Could you check a few things on this model? Use its own coordinates, in mm. A direction names the side the tool comes from. Round coordinates to 2 decimals unless told otherwise and drop trailing zeros. Write each loop counter-clockwise with the first axis right and the second up, starting at its lowest first coordinate (ties: lowest second). Pieces come first, ordered by that corner, then holes.
```python
from build123d import *

# Parameters (mm, degrees)
SKETCH_1_R          = 1.5
EXTRUDE_1_DEPTH     = 3
FILLET_1_R          = 2
SKETCH_3_W          = 25.138692766
SKETCH_3_H          = 29.703861026
CUT_EXTRUDE_1_DEPTH = 38.353045391
SKETCH_4_W          = 21
SKETCH_4_H          = 34
EXTRUDE_2_DEPTH     = 3
SKETCH_5_W          = 7
SKETCH_5_H          = 54
CUT_EXTRUDE_2_DEPTH = 50.226517244
FILLET_2_R          = 1


with BuildPart() as part:
    # 草图1 → 凸台-拉伸1 (new body)
    with BuildSketch(Plane.XY):
        Polygon((-10.5, 14), (10.5, 14), (10.5, 4), (34.5, 4), (34.5, -4), (10.5, -4), (10.5, -14), (-10.5, -14), align=None)
        with Locations((-7.5, 5)):
            Circle(SKETCH_1_R, mode=Mode.SUBTRACT)
        with Locations((7.5, 5)):
            Circle(SKETCH_1_R, mode=Mode.SUBTRACT)
        with Locations((-7.5, -5)):
            Circle(SKETCH_1_R, mode=Mode.SUBTRACT)
        with Locations((7.5, -5)):
            Circle(SKETCH_1_R, mode=Mode.SUBTRACT)
        with Locations((16.5, 0)):
            Circle(SKETCH_1_R, mode=Mode.SUBTRACT)
        with Locations((31.5, 0)):
            Circle(SKETCH_1_R, mode=Mode.SUBTRACT)
    extrude(amount=EXTRUDE_1_DEPTH)

    # 圆角1
    fillet_1_edges = [part.edges().sort_by_distance(p)[0] for p in [
        (10.5, 4, 1.5),
        (10.5, -4, 1.5),
    ]]
    fillet(fillet_1_edges, radius=FILLET_1_R)

    # 草图3 → 切除-拉伸1 (cut, through all)
    with BuildSketch(Plane.XY.offset(3)):
        with Locations((23.069346383, -0.851930513)):
            Rectangle(SKETCH_3_W, SKETCH_3_H)
    extrude(amount=-CUT_EXTRUDE_1_DEPTH, mode=Mode.SUBTRACT)

    # 草图4 → 凸台-拉伸2 (add)
    with BuildSketch(Plane.XY.offset(3)):
        with Locations((0, 31)):
            Rectangle(SKETCH_4_W, SKETCH_4_H)
    extrude(amount=-EXTRUDE_2_DEPTH)

    # 草图5 → 切除-拉伸2 (cut, through all)
    with BuildSketch(Plane.XY.offset(3)):
        with Locations((0, 17)):
            Rectangle(SKETCH_5_W, SKETCH_5_H)
    extrude(amount=-CUT_EXTRUDE_2_DEPTH, mode=Mode.SUBTRACT)

    # 圆角2
    fillet_2_edges = [part.edges().sort_by_distance(p)[0] for p in [
        (-3.5, -10, 1.5),
        (-3.5, 44, 1.5),
        (3.5, 44, 1.5),
        (3.5, -10, 1.5),
    ]]
    fillet(fillet_2_edges, radius=FILLET_2_R)


solid = part.part
```
Q1. Imagine slicing it at D-D, the plane y = 28. Write out the boundary of the cut face in (x, z).
Q2. We'd pull the mould along X, two halves only. Please class faces 1 (the cylindrical face through (3.215, 43.699, 1.479)), 2 (the flat face through (-10.5, 17, 2)), 3 (the flat face through (10.5, 17, 2)): pulls with the +X half, pulls with the -X half, needs draft (parallel to the pull), parting line crosses it, or undercut.
Q3. Imagine slicing it at A-A, the plane y = -5. Write out the boundary of the cut face in (x, z).
Q4. On a 3-axis mill with a long thin cutter (end or side, diameter ignored), from which of +Z, -Z, +X, -X, +Y, -Y can I reach the whole of each face in a straight line? I mean faces 4 (the flat face through (-5, 17, 0)), 5 (the flat face through (0, 44, 2)). Say none if no direction works.
Q5. Imagine slicing it at C-C, the plane x = 7.5. Write out the boundary of the cut face in (y, z), then the cut area to 3 significant figures.
Q6. If I drill on L1, parallel to Y at x = 7.5, z = 2.8; L2, parallel to X at y = 7, z = 1.75; L3, parallel to Y at x = 2.5, z = 2.5, over which ranges is the centre line in solid material (lowest first)?
Q7. Imagine slicing it at B-B, the plane z = 0.55. Write out the boundary of the cut face in (x, y), then the cut area to 3 significant figures.
Results found:
1. outline: (-10.5, 0) - (-3.5, 0) - (-3.5, 3) - (-10.5, 3) - close; (3.5, 0) - (10.5, 0) - (10.5, 3) - (3.5, 3) - close
2. face 1: undercut
2. face 2: pulls with the -X half
2. face 3: pulls with the +X half
3. outline: (-10.5, 0) - (-9, 0) - (-9, 3) - (-10.5, 3) - close; (-6, 0) - (-3.5, 0) - (-3.5, 3) - (-6, 3) - close; (3.5, 0) - (6, 0) - (6, 3) - (3.5, 3) - close; (9, 0) - (10.5, 0) - (10.5, 3) - (9, 3) - close
4. face 4: -Z, +X, -X, +Y, -Y
4. face 5: +Z, -Z
5. outline: (-14, 0) - (-6.5, 0) - (-6.5, 3) - (-14, 3) - close; (-3.5, 0) - (3.5, 0) - (3.5, 3) - (-3.5, 3) - close; (6.5, 0) - (48, 0) - (48, 3) - (6.5, 3) - close
5. area: 168 mm2
6. L1: y = -14 to -6.5, -3.5 to 3.5, 6.5 to 48
6. L2: x = -10.5 to -3.5, 3.5 to 10.5
6. L3: y = -14 to -10, 44 to 48
7. outline: (-10.5, -14) - (10.5, -14) - (10.5, 48) - (-10.5, 48) - close; hole circle Ø3 at (-7.5, -5); hole circle Ø3 at (-7.5, 5); hole (-3.5, -9) arc R1 ccw to (-2.5, -10) - (2.5, -10) arc R1 ccw to (3.5, -9) - (3.5, 43) arc R1 ccw to (2.5, 44) - (-2.5, 44) arc R1 ccw to (-3.5, 43) - close; hole circle Ø3 at (7.5, -5); hole circle Ø3 at (7.5, 5)
7. area: 897 mm2
